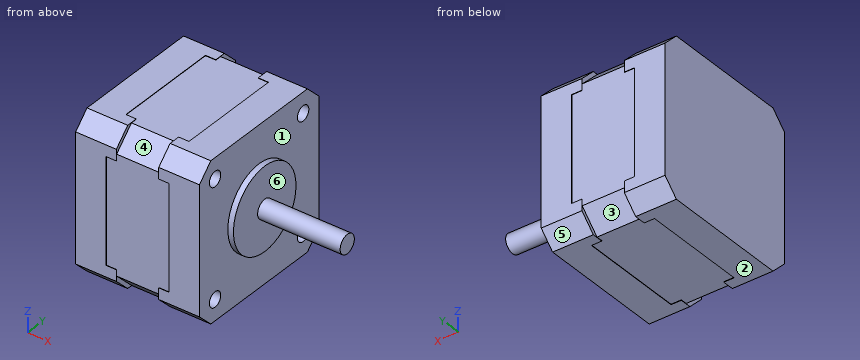
from build123d import *

# Parameters (mm, degrees)
CROQUIS1_W                  = 41.8
CROQUIS1_H                  = 41.8
SALIENTE_EXTRUIR1_DEPTH     = 11.3
CROQUIS2_W                  = 42
CROQUIS2_H                  = 41.9
SALIENTE_EXTRUIR2_DEPTH     = 10.85
CROQUIS3_W                  = 10.85
CROQUIS3_H                  = 42
SALIENTE_EXTRUIR3_DEPTH     = 0.1
CROQUIS4_W                  = 42
CROQUIS4_H                  = 42
SALIENTE_EXTRUIR4_DEPTH     = 10.85
CORTAR_EXTRUIR1_REACH       = 26.9
CROQUIS5_W                  = 0.1
CROQUIS5_H                  = 28
CORTAR_EXTRUIR2_REACH       = 26.9
CROQUIS6_W                  = 28
CROQUIS6_H                  = 0.1
CROQUIS7_W                  = 2.75
CROQUIS7_H                  = 28
CORTAR_EXTRUIR3_DEPTH       = 0.1
CROQUIS8_W                  = 2.75
CROQUIS8_H                  = 28
CORTAR_EXTRUIR4_DEPTH       = 0.1
CROQUIS9_W                  = 28
CROQUIS9_H                  = 0.1
CORTAR_EXTRUIR5_DEPTH       = 2.75
CROQUIS10_W                 = 2.75
CROQUIS10_H                 = 28
CORTAR_EXTRUIR6_DEPTH       = 0.1
CROQUIS11_W                 = 2.75
CROQUIS11_H                 = 28
CORTAR_EXTRUIR7_DEPTH       = 0.1
CROQUIS12_W                 = 2.75
CROQUIS12_H                 = 28
CORTAR_EXTRUIR8_DEPTH       = 0.1
CHAFL_N1_SIZE               = 5.214213562
CHAFL_N2_SIZE               = 4
CROQUIS18_R                 = 2
CORTAR_EXTRUIR10_DEPTH      = 6
CORTAR_EXTRUIR10_DEPTH_BACK = 3


with BuildPart() as part:
    # Croquis1 → Saliente-Extruir1 (new body)
    with BuildSketch(Plane(origin=(-5.65, 0, 0), x_dir=(0, -1, 0), z_dir=(-1, 0, 0))):
        Rectangle(CROQUIS1_W, CROQUIS1_H)
    extrude(amount=-SALIENTE_EXTRUIR1_DEPTH)

    # Croquis2 → Saliente-Extruir2 (add)
    with BuildSketch(Plane(origin=(5.65, 0, 0), x_dir=(0, 0, -1), z_dir=(1, 0, 0))):
        with Locations((0, -0.05)):
            Rectangle(CROQUIS2_W, CROQUIS2_H)
    extrude(amount=SALIENTE_EXTRUIR2_DEPTH)

    # Croquis3 → Saliente-Extruir3 (add)
    with BuildSketch(Plane(origin=(0, 20.9, 0), x_dir=(-1, 0, 0), z_dir=(0, 1, 0))):
        with Locations((-11.075, 0)):
            Rectangle(CROQUIS3_W, CROQUIS3_H)
    extrude(amount=SALIENTE_EXTRUIR3_DEPTH)

    # Croquis4 → Saliente-Extruir4 (add)
    with BuildSketch(Plane(origin=(-5.65, 0, 0), x_dir=(0, 0, -1), z_dir=(1, 0, 0))):
        Rectangle(CROQUIS4_W, CROQUIS4_H)
    extrude(amount=-SALIENTE_EXTRUIR4_DEPTH)

    # Croquis5 → Cortar-Extruir1 (cut, up to next)
    with BuildSketch(Plane(origin=(8.4, 0, 0), x_dir=(0, 0, -1), z_dir=(1, 0, 0)), mode=Mode.PRIVATE) as cortar_extruir1_sk1:
        with Locations((20.95, 0)):
            Rectangle(CROQUIS5_W, CROQUIS5_H)
    cortar_extruir1_tool1 = extrude(cortar_extruir1_sk1.sketch, amount=-CORTAR_EXTRUIR1_REACH, mode=Mode.PRIVATE) & part.part
    add(cortar_extruir1_tool1.solids().sort_by_distance((8.4, 0, -20.95))[0], mode=Mode.SUBTRACT)

    # Croquis6 → Cortar-Extruir2 (cut, up to next)
    with BuildSketch(Plane(origin=(-8.4, 0, 0), x_dir=(0, -1, 0), z_dir=(-1, 0, 0)), mode=Mode.PRIVATE) as cortar_extruir2_sk1:
        with Locations((0, 20.95)):
            Rectangle(CROQUIS6_W, CROQUIS6_H)
    cortar_extruir2_tool1 = extrude(cortar_extruir2_sk1.sketch, amount=-CORTAR_EXTRUIR2_REACH, mode=Mode.PRIVATE) & part.part
    add(cortar_extruir2_tool1.solids().sort_by_distance((-8.4, 0, 20.95))[0], mode=Mode.SUBTRACT)

    # Croquis7 → Cortar-Extruir3 (cut)
    with BuildSketch(Plane.XZ.offset(21)):
        with Locations((7.025, 0)):
            Rectangle(CROQUIS7_W, CROQUIS7_H)
    extrude(amount=-CORTAR_EXTRUIR3_DEPTH, mode=Mode.SUBTRACT)

    # Croquis8 → Cortar-Extruir4 (cut)
    with BuildSketch(Plane.XY.offset(21)):
        with Locations((7.025, 0)):
            Rectangle(CROQUIS8_W, CROQUIS8_H)
    extrude(amount=-CORTAR_EXTRUIR4_DEPTH, mode=Mode.SUBTRACT)

    # Croquis9 → Cortar-Extruir5 (cut)
    with BuildSketch(Plane.ZY.offset(-5.65)):
        with Locations((0, 20.95)):
            Rectangle(CROQUIS9_W, CROQUIS9_H)
    extrude(amount=-CORTAR_EXTRUIR5_DEPTH, mode=Mode.SUBTRACT)

    # Croquis10 → Cortar-Extruir6 (cut)
    with BuildSketch(Plane.XZ.offset(21)):
        with Locations((-7.025, 0)):
            Rectangle(CROQUIS10_W, CROQUIS10_H)
    extrude(amount=-CORTAR_EXTRUIR6_DEPTH, mode=Mode.SUBTRACT)

    # Croquis11 → Cortar-Extruir7 (cut)
    with BuildSketch(Plane(origin=(0, 0, -21), x_dir=(-1, 0, 0), z_dir=(0, 0, -1))):
        with Locations((7.025, 0)):
            Rectangle(CROQUIS11_W, CROQUIS11_H)
    extrude(amount=-CORTAR_EXTRUIR7_DEPTH, mode=Mode.SUBTRACT)

    # Croquis12 → Cortar-Extruir8 (cut)
    with BuildSketch(Plane(origin=(0, 21, 0), x_dir=(-1, 0, 0), z_dir=(0, 1, 0))):
        with Locations((7.025, 0)):
            Rectangle(CROQUIS12_W, CROQUIS12_H)
    extrude(amount=-CORTAR_EXTRUIR8_DEPTH, mode=Mode.SUBTRACT)

    # Croquis15 → Revolución1 (revolve)
    with BuildSketch(Plane.XY):
        Polygon((15.5, 11), (15.5, 0), (40, 0), (40, 2.5), (18, 2.5), (18, 11), align=None)
    revolve(axis=Axis((15.5, 0, 0), (1, 0, 0)))

    # Chaflán1
    chafl_n1_edges = [part.edges().sort_by_distance(p)[0] for p in [
        (0, -20.9, -20.9),
        (0, 20.9, 20.9),
        (0, 20.9, -20.9),
        (0, -20.9, 20.9),
    ]]
    chamfer(chafl_n1_edges, length=CHAFL_N1_SIZE)

    # Chaflán2
    chafl_n2_edges = [part.edges().sort_by_distance(p)[0] for p in [
        (11.075, -21, 21),
        (11.075, -21, -21),
        (11.075, 21, 21),
        (11.075, 21, -21),
        (-11.075, 21, -21),
        (-11.075, -21, -21),
        (-11.075, -21, 21),
        (-11.075, 21, 21),
    ]]
    chamfer(chafl_n2_edges, length=CHAFL_N2_SIZE)

    # Croquis18 → Cortar-Extruir10 (cut, two sides)
    with BuildSketch(Plane(origin=(12.45, 0, 0), x_dir=(0, 0, -1), z_dir=(1, 0, 0))) as cortar_extruir10_sk:
        with Locations((-15.5, 15.5)):
            Circle(CROQUIS18_R)
        with Locations((15.5, 15.5)):
            Circle(CROQUIS18_R)
        with Locations((15.5, -15.5)):
            Circle(CROQUIS18_R)
        with Locations((-15.5, -15.5)):
            Circle(CROQUIS18_R)
    extrude(amount=CORTAR_EXTRUIR10_DEPTH, mode=Mode.SUBTRACT)
    extrude(cortar_extruir10_sk.sketch, amount=-CORTAR_EXTRUIR10_DEPTH_BACK, mode=Mode.SUBTRACT)


solid = part.part
The model under review builds one solid part; all positions refer to its coordinate system, in mm. Face numbers are marked on the shaded views. A direction names the side the tool comes from. Coordinates: 2 decimals unless noted, no trailing zeros. Write each loop counter-clockwise with the first axis right and the second up, starting at its lowest first coordinate (ties: lowest second). Pieces come first, ordered by that corner, then holes. Notation, with made-up numbers: (87.25, -11) - (121.25, -11) arc R17 ccw to (121.25, -1) - close; hole circle Ø9 at (27.5, 5). An arc over 180 degrees is marked (long way). Answer as CSV lines item,"result".
(1) We need section C-C (x = -10.5). Give the boundary of the cut face in (y, z).
Data:
outline,"(-21, -17) - (-17, -21) - (17, -21) - (21, -17) - (21, 17) - (17, 21) - (-17, 21) - (-21, 17) - close"
(2) We need section B-B (z = -12). Give the boundary of the cut face in (x, y), plus the area to 3 significant figures.
Data:
outline,"(-16.5, -21) - (-8.4, -21) - (-8.4, -20.9) - (8.4, -20.9) - (8.4, -21) - (16.5, -21) - (16.5, 21) - (8.4, 21) - (8.4, 20.9) - (-8.4, 20.9) - (-8.4, 21) - (-16.5, 21) - close"
area,"1,380 mm2"
(3) We need section D-D (y = 0). Give the boundary of the cut face in (x, z).
Data:
outline,"(-16.5, -21) - (-8.4, -21) - (-8.4, -20.9) - (8.4, -20.9) - (8.4, -21) - (16.5, -21) - (16.5, -11) - (18, -11) - (18, -2.5) - (40, -2.5) - (40, 2.5) - (18, 2.5) - (18, 11) - (16.5, 11) - (16.5, 21) - (8.4, 21) - (8.4, 20.9) - (-8.4, 20.9) - (-8.4, 21) - (-16.5, 21) - close"
(4) Mouldability with a two-part tool opening along X and no side actions: class the marked faces 4, 5 and 6 as pulls with the +X half, pulls with the -X half, needs draft (parallel to the pull), parting line crosses it, or undercut.
Data:
face 4,"undercut"
face 5,"needs draft"
face 6,"pulls with the +X half"
(5) For line 1 along Z through (x, y) = (14.5, 15.5); line 2 along Y through (x, z) = (14, -15), list the stretches that pass through material, from the lowest coordinate up. Write a range as [from, to].
Data:
line 1,"z = [-21, -17.5], [-13.5, 13.5], [17.5, 21]"
line 2,"y = [-21, -17.44], [-13.56, 13.56], [17.44, 21]"
(6) Tool access review of the marked faces 1, 2 and 3: name each direction out of +Z, -Z, +X, -X, +Y, -Y from which nothing blocks a thin tool from reaching the whole face with its end or side.
Data:
face 1,"+X"
face 2,"-Z, +X, -X, +Y, -Y"
face 3,"-Z, +Y"
(7) We need section A-A (x = 11). Give the boundary of the cut face in (y, z), plus the area to 3 significant figures.
Data:
outline,"(-21, -17) - (-17, -21) - (17, -21) - (21, -17) - (21, 17) - (17, 21) - (-17, 21) - (-21, 17) - close; hole circle Ø4 at (-15.5, -15.5); hole circle Ø4 at (-15.5, 15.5); hole circle Ø4 at (15.5, -15.5); hole circle Ø4 at (15.5, 15.5)"
area,"1,680 mm2"
(8) Clearance check with flat-ended pins moving along their axes: pin 1 Ø13.5 at (x, y) = (-1, -4) entering from -Z; pin 2 Ø5 at (x, z) = (0, 5) entering from -Y; pin 3 Ø5 at (y, z) = (15.5, -15.5) entering from +X. State where each tip first meets the part, or that it passes through.
Data:
pin 1,"stops at z = -20.9"
pin 2,"stops at y = -20.9"
pin 3,"stops at x = 16.5"
